```python
from build123d import *

# Parameters (mm, degrees)
BOSS_EXTRUDE1_DEPTH = 45.5
SKETCH2_W           = 57.548
SKETCH2_H           = 4.628
BOSS_EXTRUDE2_DEPTH = 1.27
BOSS_EXTRUDE3_DEPTH = 38.1
CHAMFER2_SIZE       = 33.02
CHAMFER2_SIZE2      = 40.776304109
FILLET2_R           = 15.24
FILLET3_R           = 15.24


with BuildPart() as part:
    # Sketch1 → Boss-Extrude1 (new body)
    with BuildSketch(Plane.XZ.offset(154.681799526)):
        Polygon((108.516, 1.834), (107.246, 1.834), (107.246, -0.254), (146.442611067, -0.254), (162.254, -0.254), (162.254, 1.834), (160.252914004, 1.834), (160.252914004, 3.104), (163.524, 3.104), (163.524, -1.524), (105.976, -1.524), (105.976, 3.104), (108.516, 3.104), align=None)
    extrude(amount=-BOSS_EXTRUDE1_DEPTH)

    # Sketch2 → Boss-Extrude2 (add)
    with BuildSketch(Plane.XZ.offset(154.681799526)):
        with Locations((134.75, 0.79)):
            Rectangle(SKETCH2_W, SKETCH2_H)
    extrude(amount=BOSS_EXTRUDE2_DEPTH)

    # Sketch8 → Boss-Extrude3 (add)
    with BuildSketch(Plane.XY.offset(3.104)):
        Polygon((105.976, -109.181799526), (107.246, -109.181799526), (107.246, -154.681799526), (162.254, -154.681799526), (162.254, -109.181799526), (163.524, -109.181799526), (163.524, -155.951799526), (105.976, -155.951799526), align=None)
    extrude(amount=BOSS_EXTRUDE3_DEPTH)

    # Chamfer2
    chamfer2_edges = [part.edges().sort_by_distance(p)[0] for p in [
        (162.889, -109.181799526, 41.204),
        (106.611, -109.181799526, 41.204),
    ]]
    chamfer2_side = [part.faces().sort_by_distance(p)[0] for p in [
        (107.881, -109.181799526, 2.550760371),
    ]]
    chamfer(chamfer2_edges, length=CHAMFER2_SIZE, length2=CHAMFER2_SIZE2, reference=chamfer2_side[0])

    # Fillet2
    fillet2_edges = [part.edges().sort_by_distance(p)[0] for p in [
        (162.889, -109.181799526, 8.184),
        (106.611, -109.181799526, 8.184),
    ]]
    fillet(fillet2_edges, radius=FILLET2_R)

    # Fillet3
    fillet3_edges = [part.edges().sort_by_distance(p)[0] for p in [
        (106.611, -149.958103635, 41.204),
    ]]
    fillet(fillet3_edges, radius=FILLET3_R)


solid = part.part
```
The model under review builds one solid part; all positions refer to its coordinate system, in mm. A direction names the side the tool comes from. Give positions to 0.01 mm unless a question says otherwise; leave off trailing zeros. Loops run counter-clockwise (first coordinate to the right, second up) from the corner with the lowest first, then second, coordinate; pieces in that order, holes last. Notation, with made-up numbers: (45.25, -11.5) - (81.25, -11.5) arc R26 cw to (81.25, 5.5) - close; hole circle Ø6 at (16.5, 9). An arc over 180 degrees is marked (long way). Answer as a JSON object with one key per item and string values.
Q1. Add section C-C on z = 36. State the section outline as (x, y) points.
Worked out:
{"outline": "(105.98, -155.95) - (163.52, -155.95) - (163.52, -143.53) - (162.25, -143.53) - (162.25, -154.68) - (107.25, -154.68) - (107.25, -143.53) - (105.98, -143.53) - close"}
Q2. Add section B-B on y = -131. State the section outline as (x, z) points.
Worked out:
{"outline": "(105.98, -1.52) - (163.52, -1.52) - (163.52, 25.85) - (162.25, 25.85) - (162.25, 3.1) - (160.25, 3.1) - (160.25, 1.83) - (162.25, 1.83) - (162.25, -0.25) - (107.25, -0.25) - (107.25, 1.83) - (108.52, 1.83) - (108.52, 3.1) - (107.25, 3.1) - (107.25, 25.85) - (105.98, 25.85) - close"}
Q3. To check wall thickness, follow line 1 along X through (y, z) = (-129.5, 13); line 2 along Y through (x, z) = (119.5, 23); line 3 along Z through (x, y) = (117.5, -117). State the ranges of each line that lie inside material, in increasing order.
Worked out:
{"line 1": "x = 105.98 to 107.25, 162.25 to 163.52", "line 2": "y = -155.95 to -154.68", "line 3": "z = -1.52 to -0.25"}
Q4. Add section A-A on x = 143. State the section outline as (y, z) points, plus the area to 3 significant figures.
Worked out:
{"outline": "(-155.95, -1.52) - (-109.18, -1.52) - (-109.18, -0.25) - (-154.68, -0.25) - (-154.68, 41.19) arc R15.24 ccw to (-155.35, 41.2) - (-155.95, 41.2) - close", "area": "112 mm^2"}
Q5. Add section D-D on y = -118. State the section outline as (x, z) points.
Worked out:
{"outline": "(105.98, -1.52) - (163.52, -1.52) - (163.52, 15.32) - (162.25, 15.32) - (162.25, 3.1) - (160.25, 3.1) - (160.25, 1.83) - (162.25, 1.83) - (162.25, -0.25) - (107.25, -0.25) - (107.25, 1.83) - (108.52, 1.83) - (108.52, 3.1) - (107.25, 3.1) - (107.25, 15.32) - (105.98, 15.32) - close"}
Q6. For faces 5 (the cylindrical face through (162.638, -110.626, 7.39)), 6 (the flat face through (162.254, -137, 18)), 7 (the flat face through (161, -132, 1.834)), list the 3-axis set-ups (+Z, -Z, +X, -X, +Y, -Y) from which the entire face can be reached by the end or side of a thin tool; tool diameter is ignored.
Worked out:
{"face 5": "+Z, +X, -X, +Y", "face 6": "+Z, +Y", "face 7": "+Y"}
Q7. Insertion check: pin 1 (1.4 mm diameter, centred on x = 108, y = -124, fed in from +Z); pin 2 (20.5 mm diameter, centred on x = 132, z = 11.5, fed in from +Y). Each pin has a flat end and moves straight along its axis. Give the tip position at first contact, or say it passes through.
Worked out:
{"pin 1": "stops at z = 3.1", "pin 2": "stops at y = -154.68"}
Q8. Mouldability with a two-part tool opening along X and no side actions: class faces 1 (the flat face through (134, -109.182, -1)), 2 (the flat face through (163.524, -137, 15)), 3 (the flat face through (162.254, -132, 1)), 4 (the flat face through (105.976, -138, 15)) as +X half, -X half, draft (parallel to the pull), parting line (faces both ways), or undercut.
Worked out:
{"face 1": "draft", "face 2": "+X half", "face 3": "undercut", "face 4": "-X half"}
